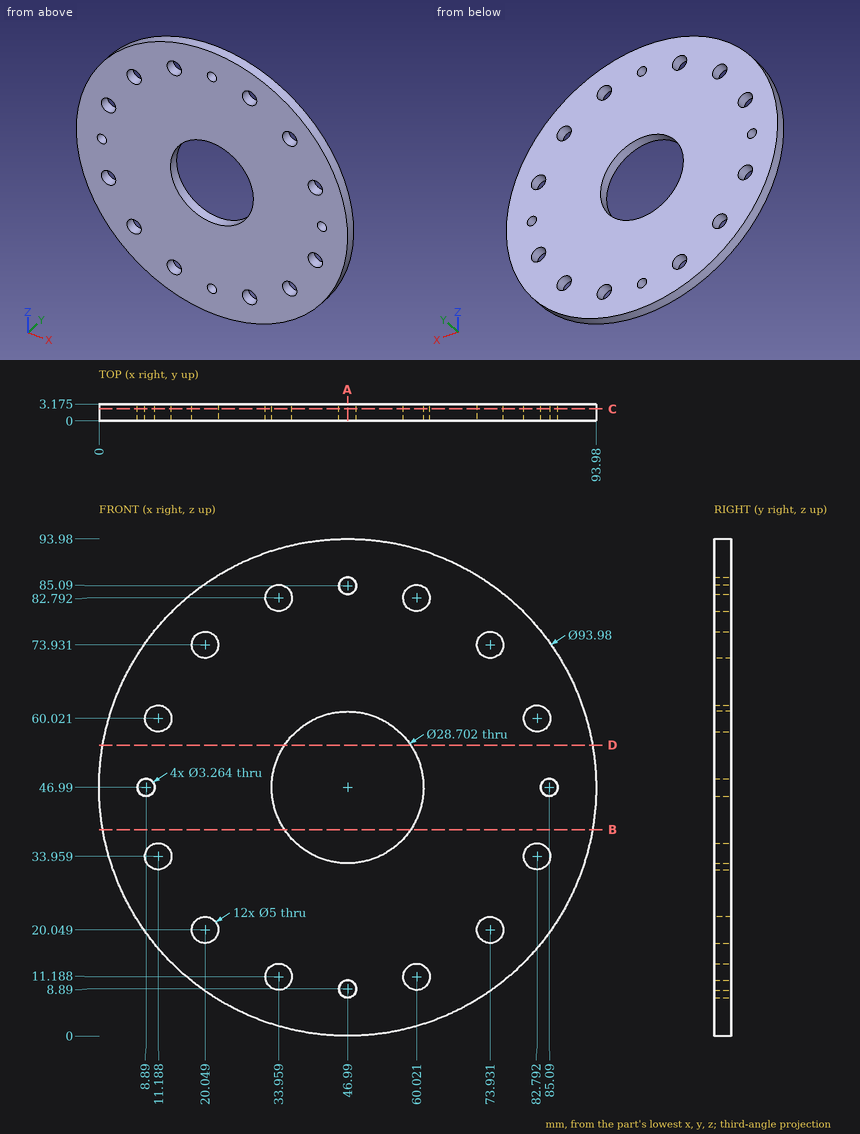
The drawing under review shows one solid part. Ordinate dimensions are in mm from its lowest x, y, z. Round coordinates to 2 decimals unless told otherwise and drop trailing zeros. Loops run counter-clockwise (first coordinate to the right, second up) from the corner with the lowest first, then second, coordinate; pieces in that order, holes last. Notation, with made-up numbers: (25, 28) - (35, 28) arc R17 cw to (35, 44) - close; hole circle Ø8 at (6, -13.5). An arc over 180 degrees is marked (long way). Put each result on its own line as item: value. Start each with the question number.
1. Consider section C-C on y = 2.25. State how many separate pieces and enclosed holes the cut face has, plus the area to 3 significant figures.
2. For probe 1 along Z at (x, y) = (13, 1.35) (1 decimal); probe 2 along Z at (x, y) = (85.09, 2.3) (1 decimal); probe 3 along Z at (x, y) = (59.5, 1.9) (1 decimal), list the stretches that pass through material, from the lowest coordinate up. Write a range as [from, to].
3. Consider section A-A on x = 46.99. State the section outline as (y, z) points (1 decimal).
4. Insertion check: P1, Ø6.5, axis at x = 20.05, z = 20.05, coming from the +Y side (3 decimals). The pin has a flat end and moves straight along its axis. Give the tip position at first contact, or say it passes through.
5. Consider section B-B on z = 39. State the section outline as (x, y) points (1 decimal).
Result sheet:
1. separate pieces: 1
1. enclosed holes: 17
1. area: 6,020 mm^2
2. probe 1: [14.5, 32.2], [35.7, 58.3], [61.7, 79.4]
2. probe 2: [19.5, 33], [34.9, 45.4], [48.6, 59], [61, 74.5]
2. probe 3: [1.7, 8.7], [13.6, 40], [54, 80.3], [85.2, 92.3]
3. outline: (0, 0) - (3.2, 0) - (3.2, 7.3) - (0, 7.3) - close; (0, 10.5) - (3.2, 10.5) - (3.2, 32.6) - (0, 32.6) - close; (0, 61.3) - (3.2, 61.3) - (3.2, 83.5) - (0, 83.5) - close; (0, 86.7) - (3.2, 86.7) - (3.2, 94) - (0, 94) - close
4. P1: y = 3.175
5. outline: (0.7, 0) - (35.1, 0) - (35.1, 3.2) - (0.7, 3.2) - close; (58.9, 0) - (93.3, 0) - (93.3, 3.2) - (58.9, 3.2) - close
